Answer from the drawing. Dimensions are ordinates in mm from the lowest x, y and z of the part. A direction names the side the tool comes from. Coordinates: 2 decimals unless noted, no trailing zeros. Order: outer loops, then holes, each group sorted by start corner. A loop starts at its lowest first (then second) coordinate and runs counter-clockwise, first axis right, second up.
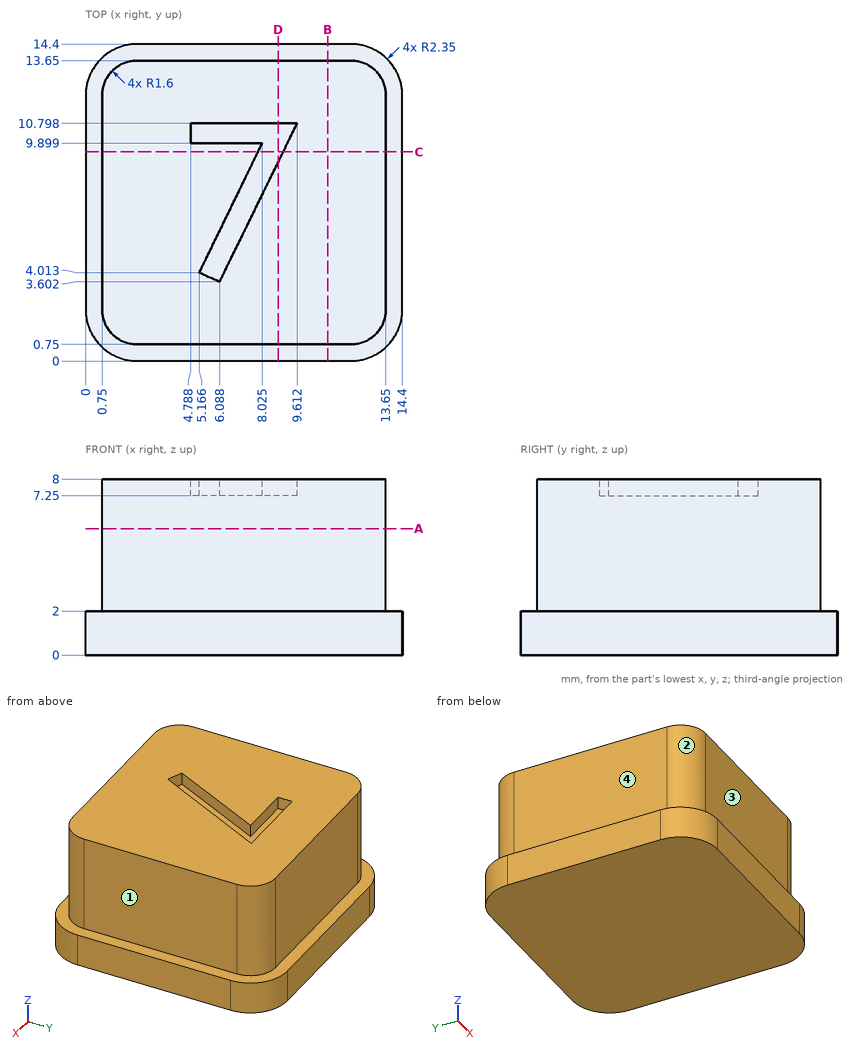
1) Section D-D (x = 8.75) is taken. Give the vertices of the cut face in (y, z), then the cut area to 3 significant figures.
2) A tool of negligible diameter and unlimited length cuts with its end or side. For the marked faces 1, 2, 3 and 4, from which of +Z, -Z, +X, -X, +Y, -Y can it reach the whole face along a straight path? Write none if from no direction.
3) Consider L1, parallel to X at y = 7, z = 6.75; L2, parallel to Z at x = 13.75, y = 3.25. Determine where each line is inside the solid, lowest interval first.
4) Each of these flat-tipped pins is pushed along its axis until it touches: P1, Ø2, axis at x = 3, z = 6, coming from the +Y side; P2, Ø1.8, axis at y = 8.5, z = 5.5, coming from the -X side; P3, Ø1.8, axis at y = 9, z = 3.5, coming from the +X side. Where does it stop, or does it pass through?
5) Section C-C (y = 9.5) is taken. Give the vertices of the cut face in (x, z).
6) Section A-A (z = 5.75) is taken. Give the vertices of the cut face in (x, y).
7) Section B-B (x = 11) is taken. Give the vertices of the cut face in (y, z), then the cut area to 3 significant figures.
Filled sheet:
1. outline: (0, 0) - (14.4, 0) - (14.4, 2) - (13.65, 2) - (13.65, 8) - (10.8, 8) - (10.8, 7.25) - (9.04, 7.25) - (9.04, 8) - (0.75, 8) - (0.75, 2) - (0, 2) - close
1. area: 105 mm2
2. face 1: +Z, +X, +Y, -Y
2. face 2: +Z, -X, -Y
2. face 3: +Z, +X, -X, -Y
2. face 4: +Z, -X, +Y, -Y
3. L1: x = 0.75 to 13.65
3. L2: z = 0 to 2
4. P1: stops at y = 13.65
4. P2: stops at x = 0.75
4. P3: stops at x = 13.65
5. outline: (0, 0) - (14.4, 0) - (14.4, 2) - (13.65, 2) - (13.65, 8) - (8.98, 8) - (8.98, 7.25) - (7.83, 7.25) - (7.83, 8) - (0.75, 8) - (0.75, 2) - (0, 2) - close
6. outline: (0.75, 2.35) arc R1.6 ccw to (2.35, 0.75) - (12.05, 0.75) arc R1.6 ccw to (13.65, 2.35) - (13.65, 12.05) arc R1.6 ccw to (12.05, 13.65) - (2.35, 13.65) arc R1.6 ccw to (0.75, 12.05) - close
7. outline: (0, 0) - (14.4, 0) - (14.4, 2) - (13.65, 2) - (13.65, 8) - (0.75, 8) - (0.75, 2) - (0, 2) - close
7. area: 106 mm2
